Here's how the part is built. I have some questions about the finished solid (model axes, mm). Face numbers are marked on the shaded views. A direction names the side the tool comes from. Give positions to 0.01 mm unless a question says otherwise; leave off trailing zeros. Loops run counter-clockwise (first coordinate to the right, second up) from the corner with the lowest first, then second, coordinate; pieces in that order, holes last. Notation, with made-up numbers: (-6.5, 40) - (40.5, 40) arc R18 cw to (40.5, 64) - close; hole circle Ø2 at (82.25, 0.25). An arc over 180 degrees is marked (long way). Use one line per item in the form item = value.
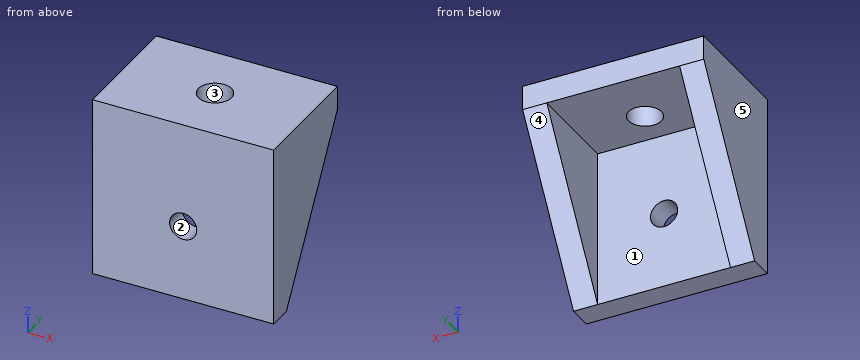
Autodesk Fusion 360 part; units mm, degrees
sketch "Sketch1" plane through (0, 0, 0) normal (0, 1, 0) x (1, 0, 0)
  line L0 (0, 0) -> (30, 0)
  line L1 (30, 0) -> (30, -30)
  line L2 (30, -30) -> (0, -30)
  line L3 (0, -30) -> (0, 0)
  dimension "d1" = 30
  dimension "d2" = 30
extrude "Extrude1" add sketch "Sketch1" along normal blind 4
sketch "Sketch2" plane through (0, 4, 0) normal (0, 1, 0) x (-1, 0, 0)
  line L0 (0, 30) -> (-30, 30)
  line L1 (-30, 30) -> (-30, 0)
  line L2 (-30, 0) -> (0, 0)
  line L3 (0, 0) -> (0, 30)
  circle A0 centre (-15, 12.5) radius 2.25
  line L4 (0, 26) -> (-30, 26)
  dimension "d5" = 4.5
  dimension "d6" = 12.5
  dimension "d7" = 15
  dimension "d23" = 4
hole "Hole1" at (15, 4, 12.5) direction (0, -1, 0) diameter 4.5 end through all
extrude "Extrude6" add sketch "Sketch2" along normal blind 16 contours L0 L1 L3 L4
sketch "Sketch7" plane through (0, 0, 30) normal (0, 0, 1) x (1, 0, 0)
  line L0 (0, 0) -> (30, 0)
  line L1 (30, 0) -> (30, 20)
  line L2 (30, 20) -> (0, 20)
  line L3 (0, 20) -> (0, 0)
  circle A0 centre (15, 10) radius 2.75
  dimension "d26" = 5.5
  dimension "d27" = 10
extrude "Extrude7" cut sketch "Sketch7" against normal through all contours A0
sketch "Sketch8" plane through (0, 0, 0) normal (-1, 0, 0) x (0, 0, 1)
  line L0 (0, 0) -> (30, 0)
  line L1 (30, 0) -> (30, 20)
  line L2 (30, 20) -> (26, 20)
  line L3 (26, 20) -> (26, 4)
  line L4 (26, 4) -> (0, 4)
  line L5 (0, 4) -> (0, 0)
  line L6 (26, 20) -> (0, 4)
extrude "Extrude8" add sketch "Sketch8" against normal blind 4 contours L3 L4 L6
sketch "Sketch9" plane through (30, 0, 0) normal (1, 0, 0) x (0, 0, -1)
  line L0 (-30, 0) -> (0, 0)
  line L1 (0, 0) -> (0, 4)
  line L2 (0, 4) -> (-26, 4)
  line L3 (-26, 4) -> (-26, 20)
  line L4 (-26, 20) -> (-30, 20)
  line L5 (-30, 20) -> (-30, 0)
  line L6 (-26, 20) -> (0, 4)
extrude "Extrude9" add sketch "Sketch9" against normal blind 4 contours L2 L3 L6
(1) For P1, Ø3, axis at x = 15.5, z = 22.5, coming from the +Y side; P2, Ø5, axis at y = 13, z = 9.5, coming from the -X side (1 decimal), each with a flat end and sliding along its axis, tell me the tip position at first contact or that it passes through.
Geometry says:
P1 = 4
P2 = through
(2) If we section it at C-C (z = 12.5): List the corners of the cut face in (x, y) for me.
Geometry says:
outline = (0, 0) - (12.75, 0) - (12.75, 4) - (4, 4) - (4, 11.69) - (0, 11.69) - close; (17.25, 0) - (30, 0) - (30, 11.69) - (26, 11.69) - (26, 4) - (17.25, 4) - close
(3) If we section it at D-D (z = 3.25): List the corners of the cut face in (x, y) for me, plus the area to 3 significant figures.
Geometry says:
outline = (0, 0) - (30, 0) - (30, 6) - (26, 6) - (26, 4) - (4, 4) - (4, 6) - (0, 6) - close
area = 136 mm²
(4) If we section it at A-A (y = 10): List the corners of the cut face in (x, z) for me.
Geometry says:
outline = (0, 9.75) - (4, 9.75) - (4, 26) - (12.25, 26) - (12.25, 30) - (0, 30) - close; (17.75, 26) - (26, 26) - (26, 9.75) - (30, 9.75) - (30, 30) - (17.75, 30) - close
(5) For the marked faces 1 and 2, which set-ups out of +Z, -Z, +X, -X, +Y, -Y let a thin tool reach every point of the face, with its end or its side?
Geometry says:
face_1 = -Z, +Y
face_2 = +Y, -Y
(6) If we section it at B-B (x = 15): List the corners of the cut face in (y, z) for me.
Geometry says:
outline = (0, 0) - (4, 0) - (4, 10.25) - (0, 10.25) - close; (0, 14.75) - (4, 14.75) - (4, 26) - (7.25, 26) - (7.25, 30) - (0, 30) - close; (12.75, 26) - (20, 26) - (20, 30) - (12.75, 30) - close
(7) If I drill on probe 1 along X at (y, z) = (5.25, 14.5); probe 2 along Z at (x, y) = (15, 1.4); probe 3 along X at (y, z) = (2.3, 12.5), over which ranges is the centre line in solid material (lowest first)?
Geometry says:
probe_1 = 0 to 4, 26 to 30
probe_2 = 0 to 10.25, 14.75 to 30
probe_3 = 0 to 12.75, 17.25 to 30
(8) Thinking about a two-plate mould opening in Y: for the marked faces 3, 4 and 5, which applies, pulls with the +Y half, pulls with the -Y half, needs draft (parallel to the pull), parting line crosses it, or undercut?
Geometry says:
face_3 = undercut
face_4 = pulls with the +Y half
face_5 = needs draft
